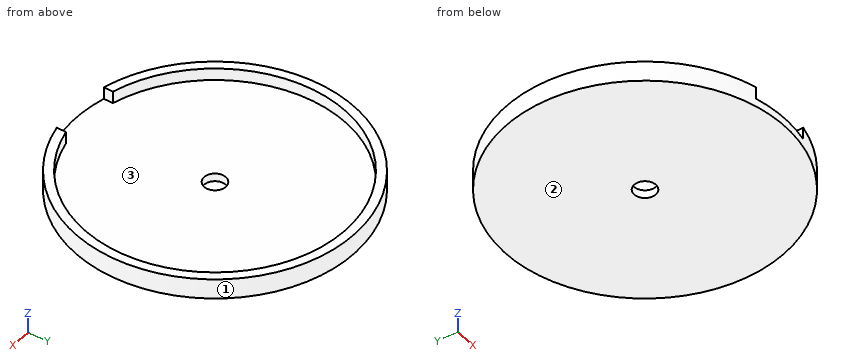
Autodesk Inventor part; units mm, degrees
ref_plane "YZ Plane" through (0, 0, 0) normal (1, 0, 0) x (0, 1, 0)
ref_plane "XZ Plane" through (0, 0, 0) normal (0, 1, 0) x (-1, 0, 0)
ref_plane "XY Plane" through (0, 0, 0) normal (0, 0, 1) x (1, 0, 0)
sketch "Skizze1" plane through (0, 0, 0) normal (0, 0, 1) x (1, 0, 0)
  circle A0 centre (0, 0) radius 34.775
  dimension "d0" = 69.55
extrude "Extrusion1" add sketch "Skizze1" along normal blind 5
sketch "Skizze2" plane through (0, 0, 5) normal (0, 0, 1) x (1, 0, 0)
  circle A0 centre (0, 0) radius 32.54
  dimension "d3" = 65.08
extrude "Extrusion2" cut sketch "Skizze2" against normal blind 3
sketch "Skizze3" plane through (0, 0, 0) normal (0, 0, -1) x (-1, 0, 0)
  circle A0 centre (0, 0) radius 2.69
  dimension "d6" = 5.38
extrude "Extrusion3" cut sketch "Skizze3" against normal through all
sketch "Skizze4" plane through (0, 0, 5) normal (0, 0, 1) x (1, 0, 0)
  line L0 (-8, -42.775) -> (8, -42.775)
  line L1 (8, -42.775) -> (8, -26.775)
  line L2 (8, -26.775) -> (-8, -26.775)
  line L3 (-8, -26.775) -> (-8, -42.775)
  circle A0 centre (0, 0) radius 34.775
  line L4 (-8, -42.775) -> (8, -26.775) construction
  line L5 (8, -42.775) -> (-8, -26.775) construction
  point P0 (0, -34.775)
  dimension "d9" = 16
  dimension "d10" = 16
extrude "Extrusion4" cut sketch "Skizze4" against normal up to surface (3 mm away) contours L3 A0 L1 L0 | L3 L2 L1 A0 picked at (0.896, -29.407)
properties part number "2024_08_28_Holder_disk_NMR"
Input: part model. Units: mm. Frame: model coordinates. Face numbers are marked on the shaded views. Coordinates: 2 decimals unless noted, no trailing zeros. Write each loop counter-clockwise with the first axis right and the second up, starting at its lowest first coordinate (ties: lowest second). Pieces come first, ordered by that corner, then holes. Notation, with made-up numbers: (-34, -2) -> (-11, -2) arc R12 ccw to (-11, 11) -> close; hole circle Ø4 at (84.5, 54). An arc over 180 degrees is marked (long way). Write each question's results on one line, items separated by ' | '.
Item 1: Section query B-B on x = 0. Return loops of the section in (y, z) (3 decimals).
Conclusion:
outline: (-34.775, 0) -> (-2.69, 0) -> (-2.69, 2) -> (-34.775, 2) -> close; (2.69, 0) -> (34.775, 0) -> (34.775, 5) -> (32.54, 5) -> (32.54, 2) -> (2.69, 2) -> close
Item 2: Section query A-A on y = 0. Return loops of the section in (x, z) (3 decimals), plus the area to 3 significant figures.
Conclusion:
outline: (-34.775, 0) -> (-2.69, 0) -> (-2.69, 2) -> (-32.54, 2) -> (-32.54, 5) -> (-34.775, 5) -> close; (2.69, 0) -> (34.775, 0) -> (34.775, 5) -> (32.54, 5) -> (32.54, 2) -> (2.69, 2) -> close | area: 142 mm^2
Item 3: Material intervals for probe 1 along X at (y, z) = (-1, 3.15); probe 2 along Y at (x, z) = (0, 1.3) (3 decimals); probe 3 along Y at (x, z) = (0, 2.9) (3 decimals), sorted ascending.
Conclusion:
probe 1: x = -34.76 to -32.52, 32.52 to 34.76 | probe 2: y = -34.775 to -2.69, 2.69 to 34.775 | probe 3: y = 32.54 to 34.775
Item 4: Section query D-D on y = 24.5. Return loops of the section in (x, z), plus the area to 3 significant figures.
Conclusion:
outline: (-24.68, 0) -> (24.68, 0) -> (24.68, 5) -> (21.41, 5) -> (21.41, 2) -> (-21.41, 2) -> (-21.41, 5) -> (-24.68, 5) -> close | area: 118 mm^2
Item 5: Mould query, pull axis Y, two halves, no side actions, for the marked faces 1, 2 and 3. Classes: +Y half, -Y half, draft (parallel to the pull), parting line (faces both ways), or undercut.
Conclusion:
face 1: parting line | face 2: draft | face 3: undercut
Item 6: Section query C-C on z = 0.95. Return loops of the section in (x, y) (3 decimals).
Conclusion:
outline: circle Ø69.55 at (0, 0); hole circle Ø5.38 at (0, 0)
Item 7: Pin query (flat end, axial travel): pin 1 Ø1.2 at (y, z) = (-32.5, 3.5) entering from -X; pin 2 Ø3 at (y, z) = (23, 4.5) entering from +X; pin 3 Ø3 at (x, z) = (-18.5, 2.5) entering from -Y; pin 4 Ø3 at (x, y) = (0, 0) entering from +Z. Return the tip coordinate at first contact, or that it passes through.
Conclusion:
pin 1: stops at x = -13.85 | pin 2: stops at x = 27.33 | pin 3: stops at y = -30.34 | pin 4: passes through
